The model under review builds one solid part; all positions refer to its coordinate system, in mm. Coordinates: 2 decimals unless noted, no trailing zeros. Loops run counter-clockwise (first coordinate to the right, second up) from the corner with the lowest first, then second, coordinate; pieces in that order, holes last. Notation, with made-up numbers: (-36, 7.25) - (-16, 7.25) arc R21 ccw to (-16, 46.25) - close; hole circle Ø4 at (2, 63). An arc over 180 degrees is marked (long way). Use a Markdown table: item, result. Add a question column.
1) Add section A-A, the plane x = 48. Give the boundary of the cut face in (y, z), and give its area (3 significant figures).
2) Clearance check with a flat-ended pin moving along its axis: pin 1 (4 mm diameter, centred on x = -8.5, z = -0.5, fed in from -Y). State where the tip first meets the part, or that it passes through.
3) Add section B-B, the plane z = -0.75. Give the boundary of the cut face in (x, y), and give its area (3 significant figures).
4) Add section C-C, the plane y = 1.3. Give the number of separate pieces and of enclosed holes in the cut face, and give its area (3 significant figures).
5) To check wall thickness, follow L1, parallel to X at y = 1.4, z = -5.25; L2, parallel to X at y = 5.25, z = -1.5; L3, parallel to Z at x = -37.5, y = 1.4. State the ranges of each line that lie inside material, in increasing order. Write a range as [from, to].
```python
from build123d import *

# Parameters (mm, degrees)
SKETCH1_W                                = 181
SKETCH1_H                                = 20
BOSS_EXTRUDE1_DEPTH                      = 6
SKETCH3_W                                = 30
SKETCH3_H                                = 6
CUT_EXTRUDE1_DEPTH                       = 7
SKETCH4_W                                = 6
SKETCH4_H                                = 5
CUT_EXTRUDE2_DEPTH                       = 7
FILLET1_R                                = 2
BOSS_EXTRUDE2_DEPTH                      = 6
MIRROR2_AT_THE_SECOND_PLANE_COPY_1_DEPTH = 6


with BuildPart() as part:
    # Sketch1 → Boss-Extrude1 (new body)
    with BuildSketch(Plane(origin=(0, 0, 0), x_dir=(1, 0, 0), z_dir=(0, 1, 0))):
        Rectangle(SKETCH1_W, SKETCH1_H)
    extrude(amount=BOSS_EXTRUDE1_DEPTH)

    # Sketch3 → Cut-Extrude1 (cut, through all)
    with BuildSketch(Plane(origin=(0, 6, 0), x_dir=(1, 0, 0), z_dir=(0, 1, 0))):
        with Locations((36, 0)):
            Rectangle(SKETCH3_W, SKETCH3_H)
        Rectangle(SKETCH3_W, SKETCH3_H)
        with Locations((-36, 0)):
            Rectangle(SKETCH3_W, SKETCH3_H)
    extrude(amount=-CUT_EXTRUDE1_DEPTH, mode=Mode.SUBTRACT)

    # Sketch4 → Cut-Extrude2 (cut, through all)
    with BuildSketch(Plane.XZ):
        with Locations((-66.7, 7.5)):
            Rectangle(SKETCH4_W, SKETCH4_H)
        with Locations((-66.7, -7.5)):
            Rectangle(SKETCH4_W, SKETCH4_H)
    cut_extrude2 = extrude(amount=-CUT_EXTRUDE2_DEPTH, mode=Mode.SUBTRACT)

    # Mirror1: Cut-Extrude2 across plane
    add(cut_extrude2.mirror(Plane(origin=(0, 0, 0), x_dir=(0, 0, 1), z_dir=(1, 0, 0))), mode=Mode.SUBTRACT)

    # Fillet1
    fillet1_edges = [part.edges().sort_by_distance(p)[0] for p in [
        (-90.5, 3, -10),
        (-90.5, 3, 10),
        (90.5, 3, 10),
        (90.5, 3, -10),
    ]]
    fillet(fillet1_edges, radius=FILLET1_R)

    # Sketch5 → Boss-Extrude2 (add)
    with BuildSketch(Plane(origin=(0, 6, 0), x_dir=(1, 0, 0), z_dir=(0, 1, 0))):
        Polygon((-69.5, 5.2), (-69.5, 9.8), (-69.5, 10), (-69.7, 10), (-69.7, 5), (-63.7, 5), (-63.7, 10), (-63.9, 10), (-63.9, 9.8), (-63.9, 5.2), align=None)
    boss_extrude2 = extrude(amount=-BOSS_EXTRUDE2_DEPTH)

    # Mirror2: Boss-Extrude2 across plane
    add(boss_extrude2.mirror(Plane(origin=(0, 0, 0), x_dir=(0, 0, 1), z_dir=(1, 0, 0))))

    # Mirror2 at the second plane: Boss-Extrude2 across plane
    add(boss_extrude2.mirror(Plane.XY))

    # Mirror2 at the second plane copy 1 sketc → Mirror2 at the second plane copy 1 (add)
    with BuildSketch(Plane(origin=(0, 6, 0), x_dir=(-1, 0, 0), z_dir=(0, 1, 0))):
        Polygon((-69.5, 5.2), (-69.5, 9.8), (-69.5, 10), (-69.7, 10), (-69.7, 5), (-63.7, 5), (-63.7, 10), (-63.9, 10), (-63.9, 9.8), (-63.9, 5.2), align=None)
    extrude(amount=-MIRROR2_AT_THE_SECOND_PLANE_COPY_1_DEPTH)


solid = part.part
```
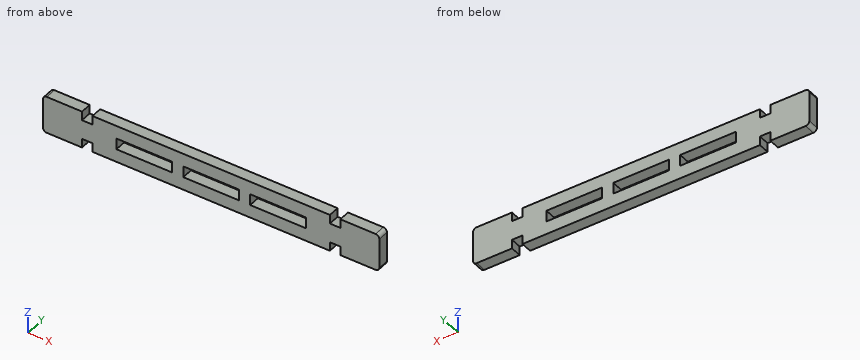
From the geometry:
| question | item | result |
|---|---|---|
| 1 | outline | (0, -10) - (6, -10) - (6, -3) - (0, -3) - close; (0, 3) - (6, 3) - (6, 10) - (0, 10) - close |
| 1 | area | 84.0 mm^2 |
| 2 | pin 1 | passes through |
| 3 | outline | (-90.5, 0) - (-51, 0) - (-51, 6) - (-90.5, 6) - close; (-21, 0) - (-15, 0) - (-15, 6) - (-21, 6) - close; (15, 0) - (21, 0) - (21, 6) - (15, 6) - close; (51, 0) - (90.5, 0) - (90.5, 6) - (51, 6) - close |
| 3 | area | 546 mm^2 |
| 4 | separate pieces | 1 |
| 4 | enclosed holes | 3 |
| 4 | area | 2,970 mm^2 |
| 5 | L1 | x = [-90.5, -69.5], [-63.9, 63.9], [69.5, 90.5] |
| 5 | L2 | x = [-90.5, -51], [-21, -15], [15, 21], [51, 90.5] |
| 5 | L3 | z = [-10, -3], [3, 10] |
